from build123d import *

# Parameters (mm, degrees)
SKETCH1_R                       = 31.5
BOSS_EXTRUDE1_DEPTH             = 11
TAP_DRILL_FOR_M3X0_5_TAP1_D     = 2.5
TAP_DRILL_FOR_M3X0_5_TAP1_DEPTH = 7
TAP_DRILL_FOR_M3X0_5_TAP1_TIP   = 0.751075774
SKETCH9_OUTSIDE_W               = 82.954
SKETCH9_OUTSIDE_H               = 82.954
SKETCH9_OUTSIDE_R               = 27
CUT_EXTRUDE1_DEPTH              = 10


with BuildPart() as part:
    # Sketch1 → Boss-Extrude1 (new body)
    with BuildSketch(Plane(origin=(0, 0, 0), x_dir=(1, 0, 0), z_dir=(0, 1, 0))):
        Circle(SKETCH1_R)
    extrude(amount=BOSS_EXTRUDE1_DEPTH)

    # Tap Drill for M3x0.5 Tap1
    with Locations(Plane(origin=(0, 11, 0), x_dir=(1, 0, 0), z_dir=(0, 1, 0))):
        with Locations((-8.838834765, 8.838834765), (8.838834765, 8.838834765), (8.838834765, -8.838834765), (-8.838834765, -8.838834765)):
            Hole(TAP_DRILL_FOR_M3X0_5_TAP1_D / 2, depth=TAP_DRILL_FOR_M3X0_5_TAP1_DEPTH)
            with Locations((0, 0, -(TAP_DRILL_FOR_M3X0_5_TAP1_DEPTH + TAP_DRILL_FOR_M3X0_5_TAP1_TIP / 2))):  # 118° drill point
                Cone(0, TAP_DRILL_FOR_M3X0_5_TAP1_D / 2, TAP_DRILL_FOR_M3X0_5_TAP1_TIP, mode=Mode.SUBTRACT)

    # Sketch9 outside → Cut-Extrude1 (cut)
    with BuildSketch(Plane.XZ):
        Rectangle(SKETCH9_OUTSIDE_W, SKETCH9_OUTSIDE_H)
        Circle(SKETCH9_OUTSIDE_R, mode=Mode.SUBTRACT)
    extrude(amount=-CUT_EXTRUDE1_DEPTH, mode=Mode.SUBTRACT)


solid = part.part
Geometry: final body of the model. Coordinates: model frame, mm. A direction names the side the tool comes from. Round coordinates to 2 decimals unless told otherwise and drop trailing zeros. Loops run counter-clockwise (first coordinate to the right, second up) from the corner with the lowest first, then second, coordinate; pieces in that order, holes last.
Q1. Section B-B on x = -14.5. Return loops of the section in (y, z), plus the area to 3 significant figures.
Q2. Material intervals for L1, parallel to Y at x = 20.5, z = 18; L2, parallel to X at y = 9, z = 8.5; L3, parallel to X at y = 2, z = -3.5, sorted ascending.
Q3. Section C-C on y = 1. Return loops of the section in (x, z), plus the area to 3 significant figures.
Q4. Section A-A on z = 0. Return loops of the section in (x, y).
Q5. Pin query (flat end, axial travel): P1, Ø6, axis at x = 14.5, y = 5.5, coming from the +Z side; P2, Ø3, axis at y = 2, z = 3, coming from the -X side; P3, Ø2, axis at x = -16, y = 3.5, coming from the +Z side. Return the tip coordinate at first contact, or that it passes through.
Q6. Access query for faces 1 (the flat face through (0, 11, 0)), 2 (the cylindrical face through (-5.85, 4.93, -26.36)), 3 (the cylindrical face through (-7.59, 7.45, 8.78)). Directions: +Z, -Z, +X, -X, +Y, -Y. A direction counts if a zero-diameter tool reaches every point of the face in a straight line with its end or side. Return the directions, or none.
Q7. Pull-direction query (Z, two-part tool) for faces 4 (the cylindrical face through (10.088, 7.451, 8.784)), 5 (the flat face through (23.19, 10, 14.15)), 6 (the cylindrical face through (-4.101, 10.493, -31.232)); classes: released by +Z, released by -Z, zero draft, split by the parting line, or undercut.
Evaluation:
1. outline: (0, -22.78) - (10, -22.78) - (10, -27.96) - (11, -27.96) - (11, 27.96) - (10, 27.96) - (10, 22.78) - (0, 22.78) - close
1. area: 511 mm2
2. L1: y = 10 to 11
2. L2: x = -25.63 to -10.04, -7.64 to 7.64, 10.04 to 25.63
2. L3: x = -26.77 to 26.77
3. outline: circle Ø54 at (0, 0)
3. area: 2,290 mm2
4. outline: (-31.5, 10) - (-27, 10) - (-27, 0) - (27, 0) - (27, 10) - (31.5, 10) - (31.5, 11) - (-31.5, 11) - close
5. P1: stops at z = 24.43
5. P2: stops at x = -26.96
5. P3: stops at z = 22.45
6. face 1: +Z, -Z, +X, -X, +Y
6. face 2: -Y
6. face 3: +Y
7. face 4: undercut
7. face 5: zero draft
7. face 6: split by the parting line
